CAD build for the part. Positions are in the model's coordinates, mm. Coordinates: 2 decimals unless noted, no trailing zeros. Write each loop counter-clockwise with the first axis right and the second up, starting at its lowest first coordinate (ties: lowest second). Pieces come first, ordered by that corner, then holes. Notation, with made-up numbers: (86, 56) - (97, 56) arc R20 cw to (97, 68) - close; hole circle Ø9 at (-28, 77). An arc over 180 degrees is marked (long way). One line per question, with ' | ' between items. Start each with the question number.
1. Flat gauge pins, fed straight in: P1, Ø5, axis at x = 190, z = 238.5, coming from the +Y side; P2, Ø1.5, axis at x = 21, y = 1, coming from the +Z side. Where does each tip first touch, or does it go through?
2. Band-saw the part on A-A, the plane y = 2.4. Give the number of separate pieces and of enclosed holes in the cut face, then the cut area to 3 significant figures.
3. Probe line 1 (X direction, y = 1, z = 358.5); line 2 (X direction, y = 1.6, z = 403.5); line 3 (X direction, y = 1.25, z = 369.5). List the from-to ranges inside material, lowest first.
4. Band-saw the part on B-B, the plane x = 94.5. Write the cut outline in (y, z).
Autodesk Inventor part; units mm, degrees
ref_plane "YZ Plane" through (0, 0, 0) normal (1, 0, 0) x (0, 1, 0)
ref_plane "XZ Plane" through (0, 0, 0) normal (0, 1, 0) x (-1, 0, 0)
ref_plane "XY Plane" through (0, 0, 0) normal (0, 0, 1) x (1, 0, 0)
sketch "Skizze1" plane through (0, 0, 0) normal (0, 1, 0) x (-1, 0, 0)
  line L0 (0, 0) -> (-698, 0)
  line L1 (-698, 0) -> (-698, 597)
  line L2 (-698, 597) -> (0, 597)
  line L3 (0, 597) -> (0, 0)
  line L4 (-349, 0) -> (-349, 597) construction
  line L5 (0, 298.5) -> (-698, 298.5) construction
  line L6 (-190, 0) -> (-190, 597) construction
  line L7 (-508, 0) -> (-508, 597) construction
  line L8 (-698, 407) -> (0, 407) construction
  line L9 (0, 80) -> (-698, 80) construction
  line L10 (-683, 582) -> (-683, 15) construction
  line L11 (-683, 15) -> (-15, 15) construction
  line L12 (-15, 15) -> (-15, 582) construction
  line L13 (-15, 582) -> (-683, 582) construction
  line L14 (-23, 362) -> (-7, 362) construction
  line L15 (-7, 362) -> (-7, 452) construction
  line L16 (-7, 452) -> (-23, 452) construction
  line L17 (-23, 452) -> (-23, 362) construction
  line L18 (-23, 362) -> (-7, 452) construction
  line L19 (-7, 362) -> (-23, 452) construction
  line L20 (-145, 590) -> (-235, 590) construction
  line L21 (-235, 590) -> (-235, 574) construction
  line L22 (-235, 574) -> (-145, 574) construction
  line L23 (-145, 574) -> (-145, 590) construction
  line L24 (-145, 590) -> (-235, 574) construction
  line L25 (-235, 590) -> (-145, 574) construction
  line L26 (-304, 590) -> (-394, 590) construction
  line L27 (-394, 590) -> (-394, 574) construction
  line L28 (-394, 574) -> (-304, 574) construction
  line L29 (-304, 574) -> (-304, 590) construction
  line L30 (-304, 590) -> (-394, 574) construction
  line L31 (-394, 590) -> (-304, 574) construction
  circle A0 centre (-15, 399.5) radius 3.25
  circle A1 centre (-15, 370) radius 4.5
  circle A2 centre (-15, 414.5) radius 3.25
  circle A3 centre (-15, 444) radius 4.5
  circle A4 centre (-182.5, 582) radius 3.25
  circle A5 centre (-153, 582) radius 4.5
  circle A6 centre (-312, 582) radius 4.5
  circle A7 centre (-341.5, 582) radius 3.25
  circle A8 centre (-197.5, 582) radius 3.25
  circle A9 centre (-227, 582) radius 4.5
  circle A10 centre (-386, 582) radius 4.5
  circle A11 centre (-356.5, 582) radius 3.25
  circle A12 centre (-683, 399.5) radius 3.25
  circle A13 centre (-683, 370) radius 4.5
  circle A14 centre (-683, 444) radius 4.5
  circle A15 centre (-683, 414.5) radius 3.25
  circle A16 centre (-515.5, 582) radius 3.25
  circle A17 centre (-545, 582) radius 4.5
  circle A18 centre (-500.5, 582) radius 3.25
  circle A19 centre (-471, 582) radius 4.5
  circle A20 centre (-15, 43) radius 4.5
  circle A21 centre (-15, 72.5) radius 3.25
  circle A22 centre (-190, 238.5) radius 2.75
  circle A23 centre (-190, 358.5) radius 2.75
  circle A24 centre (-508, 238.5) radius 2.75
  circle A25 centre (-508, 358.5) radius 2.75
  circle A26 centre (-15, 117) radius 4.5
  circle A27 centre (-15, 87.5) radius 3.25
  circle A28 centre (-683, 43) radius 4.5
  circle A29 centre (-683, 72.5) radius 3.25
  circle A30 centre (-683, 87.5) radius 3.25
  circle A31 centre (-683, 117) radius 4.5
  line L32 (0, 482) -> (-35, 482)
  line L33 (-35, 482) -> (-115, 562)
  line L34 (-115, 562) -> (-115, 597)
  line L35 (-698, 482) -> (-663, 482)
  line L36 (-663, 482) -> (-583, 562)
  line L37 (-583, 562) -> (-583, 597)
  line L38 (-328, 597) -> (-370, 597)
  line L39 (-370, 597) -> (-370, 555)
  line L40 (-370, 555) -> (-328, 555)
  line L41 (-328, 555) -> (-328, 597)
  line L42 (-328, 555) -> (-320.5943, 597)
  line L43 (-370, 555) -> (-377.4057, 597)
  point P0 (-15, 407)
  point P1 (-190, 582)
  point P2 (-349, 582)
  point P3 (-190, 298.5)
  dimension "d0" = 698
  dimension "d1" = 597
  dimension "d2" = 190
  dimension "d3" = 80
  dimension "d4" = 190
  dimension "d5" = 190
  dimension "d6" = 15
  dimension "d7" = 16
  dimension "d8" = 90
  dimension "d9" = 90
  dimension "d10" = 16
  dimension "d11" = 90
  dimension "d12" = 16
  dimension "d13" = 6.5
  dimension "d14" = 7.5
  dimension "d15" = 9
  dimension "d16" = 37
  dimension "d17" = 6.5
  dimension "d18" = 9
  dimension "d19" = 7.5
  dimension "d20" = 37
  dimension "d21" = 6.5
  dimension "d22" = 9
  dimension "d23" = 7.5
  dimension "d24" = 37
  dimension "d30" = 5.5
  dimension "d34" = 6.5
  dimension "d35" = 9
  dimension "d36" = 7.5
  dimension "d37" = 37
  dimension "d80" = 115
  dimension "d81" = 115
  dimension "d82" = 45
  dimension "d83" = 35
  dimension "d84" = 42
  dimension "d85" = 10
  dimension "d86" = 42
extrude "Ex-Platte" add sketch "Skizze1" along normal blind 3 contours L0 L1 L35 L36 L37 L2 L43 L40 L42 L34 L33 L32 L3 | A6 | A10
chamfer "Fase-15mm" distance 15 angle 45 6 edges at (698, 1.5, 0) (0, 1.5, 0) (0, 1.5, 482) (115, 1.5, 597) (583, 1.5, 597) (698, 1.5, 482)
ref_plane "Mittelebene" through (683, 0, 298.5) normal (0, 0, -1) x (-1, 0, 0)
sketch "Profil-Verstärkung" plane through (0, 0, 0) normal (0, 1, 0) x (-1, 0, 0)
  line L0 (-683, 0) -> (-15, 0)
  line L1 (0, 15) -> (0, 482)
  line L2 (-115, 597) -> (-583, 597)
  line L3 (-698, 482) -> (-698, 15)
  line L4 (0, 248.5) -> (-698, 248.5) construction
  circle A0 centre (-15, 117) radius 4.5
  circle A1 centre (-15, 370) radius 4.5
  circle A2 centre (-190, 358.5) radius 2.75
  circle A3 centre (-190, 238.5) radius 2.75
  circle A4 centre (-227, 582) radius 4.5
  line L5 (-349, 0) -> (-349, 597) construction
  circle A5 centre (-349, 298.5) radius 2.5
  circle A6 centre (-429, 298.5) radius 2.5
  circle A7 centre (-509, 298.5) radius 2.5
  circle A8 centre (-589, 298.5) radius 2.5
  circle A9 centre (-669, 298.5) radius 2.5
  circle A10 centre (-349, 323.5) radius 2.5
  circle A11 centre (-349, 403.5) radius 2.5
  circle A12 centre (-349, 483.5) radius 2.5
  circle A13 centre (-349, 563.5) radius 2.5
  circle A14 centre (-269, 298.5) radius 2.5
  circle A15 centre (-189, 298.5) radius 2.5
  circle A16 centre (-109, 298.5) radius 2.5
  circle A17 centre (-29, 298.5) radius 2.5
  line L6 (139.6, 298.5) -> (-837.6, 298.5) construction
  circle A18 centre (-349, 273.5) radius 2.5
  circle A19 centre (-349, 193.5) radius 2.5
  circle A20 centre (-349, 113.5) radius 2.5
  circle A21 centre (-349, 33.5) radius 2.5
  point P0 (0, 0)
  dimension "d38" = 698
  dimension "d40" = 121.5
  dimension "d42" = 11.5
  dimension "d61" = 5
  dimension "d64" = 80
  dimension "d69" = 5
  dimension "d70" = 25
  dimension "d73" = 80
extrude "Ex-ProfilBohrungen" cut sketch "Profil-Verstärkung" along normal up to surface (3 mm away) contours A5 | A6 | A7 | A8 | A9 | A10 | A11 | A12 | A13 | A14 | A15 | A16 | A17 | A18 | A19 | A20 | A21
fillet "Rundung-2mm" radius 2 4 edges at (370, 1.5, 555) (328, 1.5, 555) (320.5943, 1.5, 597) (377.4057, 1.5, 597)
equation "\"d5\" = d4"
equation "\"d17\" = d13"
equation "\"d18\" = d15"
equation "\"d19\" = d14"
equation "\"d20\" = d16"
equation "\"d21\" = d13"
equation "\"d22\" = d15"
equation "\"d23\" = d14"
equation "\"d24\" = d16"
equation "\"d34\" = d13"
equation "\"d35\" = d15"
equation "\"d36\" = d14"
equation "\"d37\" = d16"
equation "\"d81\" = d80"
equation "\"d69\" = d61"
properties part number "enc-SidePanel Unten V2 596x698"
Filled in:
1) P1: passes through | P2: stops at z = 482
2) separate pieces: 1 | enclosed holes: 44 | area: 392,000 mm²
3) line 1: x = 0 to 187.25, 192.75 to 505.25, 510.75 to 698 | line 2: x = 0 to 346.5, 351.5 to 698 | line 3: x = 0 to 10.53, 19.47 to 678.53, 687.47 to 698
4) outline: (0, 0) - (3, 0) - (3, 541.5) - (0, 541.5) - close
